from build123d import *

# Parameters (mm, degrees)
F0_W     = 101.6
F0_H     = 76.2
F1_DEPTH = 63.5
F3_DEPTH = 127
F4_W     = 50.8
F4_H     = 38.1
F5_DEPTH = 57.15


with BuildPart() as f1:
    # F0 (on Front) → F1 (new body)
    with BuildSketch(Plane.XZ):
        with Locations((5.107021, 0.342115)):
            Rectangle(F0_W, F0_H)
    extrude(amount=F1_DEPTH)

    # F2 (on face) → F3 (cut)
    with BuildSketch(Plane(origin=(-45.692979, 0, 0), x_dir=(0, -1, 0), z_dir=(-1, 0, 0))):
        with BuildLine():
            ThreePointArc((12.7, 38.442115), (27.598959, 2.541074), (63.5, -12.357885))
            Line((63.5, -12.357885), (63.5, 38.442115))
            Line((63.5, 38.442115), (12.7, 38.442115))
        make_face()
    extrude(amount=-F3_DEPTH, mode=Mode.SUBTRACT)

    # F4 (on face) → F5 (cut)
    with BuildSketch(Plane(origin=(0, 0, 0), x_dir=(-1, 0, 0), z_dir=(0, 1, 0))):
        with Locations((-5.107021, 19.392115)):
            Rectangle(F4_W, F4_H)
    extrude(amount=-F5_DEPTH, mode=Mode.SUBTRACT)


solid = f1.part
The model under review builds one solid part; all positions refer to its coordinate system, in mm. A direction names the side the tool comes from. Give positions to 0.01 mm unless a question says otherwise; leave off trailing zeros. Write each loop counter-clockwise with the first axis right and the second up, starting at its lowest first coordinate (ties: lowest second). Pieces come first, ordered by that corner, then holes. Notation, with made-up numbers: M 37,-29.75 L 48,-29.75 A12 ccw 48,-6.75 Z; hole C -33.75,62.5 d3. An arc over 180 degrees is marked long. One line per question, with ' | ' between items. Start each with the question number.
Item 1: Wall thickness on line 1 (X direction, y = -8.5, z = 15.5); line 2 (Z direction, x = 6, y = -19.5); line 3 (Z direction, x = -6, y = -46): over which ranges is each line inside the solid? List them lowest first. Write a range as from..to.
Item 2: Draft analysis for pull direction X (two halves, no side actions). For faces 1 (the flat face through (-45.693, -24, -9)), 2 (the flat face through (30.507, -8, 15)), 3 (the flat face through (4, 0, -8)), state which applies: released by +X, released by -X, zero draft, split by the parting line, or undercut.
Item 3: We need section B-B on x = 10.5. Write out the cut boundary in (y, z), plus the area to 3 significant figures.
Item 4: We need section D-D on z = 31.5. Write out the cut boundary in (x, y).
Item 5: We need section C-C on y = -17.5. Write out the cut boundary in (x, z).
Item 6: For pin 1 (1 mm diameter, centred on x = 33.5, y = -32.5, fed in from +Z); pin 2 (1.5 mm diameter, centred on x = 12, y = -28.5, fed in from +Z); pin 3 (5 mm diameter, centred on x = -32.5, z = 15.5, fed in from -Y), all flat-tipped, find the tip position at first contact; note any pin that passes through.
Item 7: For faces 4 (the flat face through (-20.293, -8, 15)), 5 (the flat face through (-33, -6, 38.442)), list the 3-axis set-ups (+Z, -Z, +X, -X, +Y, -Y) from which the entire face can be reached by the end or side of a thin tool; tool diameter is ignored.
Item 8: We need section A-A on z = 18.5. Write out the cut boundary in (x, y).
Results found:
1) line 1: x = -45.69..-20.29, 30.51..55.91 | line 2: z = -37.76..0.34 | line 3: z = -37.76..-9.23
2) face 1: released by -X | face 2: undercut | face 3: zero draft
3) outline: M -63.5,-37.76 L 0,-37.76 L 0,0.34 L -29.94,0.34 A50.87 cw -63.5,-12.36 Z | area: 2,130 mm2
4) outline: M -45.69,-13.19 L -20.29,-13.19 L -20.29,0 L -45.69,0 Z; M 30.51,-13.19 L 55.91,-13.19 L 55.91,0 L 30.51,0 Z
5) outline: M -45.69,-37.76 L 55.91,-37.76 L 55.91,16.94 L 30.51,16.94 L 30.51,0.34 L -20.29,0.34 L -20.29,16.94 L -45.69,16.94 Z
6) pin 1: stops at z = -1.38 | pin 2: stops at z = 0.34 | pin 3: stops at y = -19.56
7) face 4: +Z, +Y, -Y | face 5: +Z, +X, -X, +Y, -Y
8) outline: M -45.69,-16.8 L -20.29,-16.8 L -20.29,0 L -45.69,0 Z; M 30.51,-16.8 L 55.91,-16.8 L 55.91,0 L 30.51,0 Z
